The model under review builds one solid part; all positions refer to its coordinate system, in mm. A direction names the side the tool comes from. Coordinates: 2 decimals unless noted, no trailing zeros. Order: outer loops, then holes, each group sorted by start corner. A loop starts at its lowest first (then second) coordinate and runs counter-clockwise, first axis right, second up. Notation, with made-up numbers: M -34.5,-22 L -25.5,-22 A8 cw -25.5,-16 Z; hole C 26.5,67.5 d3. An arc over 180 degrees is marked long. Answer in a Markdown table with one row per item.
Autodesk Inventor part; units mm, degrees
ref_plane "YZ Plane" through (0, 0, 0) normal (1, 0, 0) x (0, 1, 0)
ref_plane "XZ Plane" through (0, 0, 0) normal (0, 1, 0) x (-1, 0, 0)
ref_plane "XY Plane" through (0, 0, 0) normal (0, 0, 1) x (1, 0, 0)
sketch "Boceto1" plane through (0, 0, 0) normal (0, 1, 0) x (-1, 0, 0)
  circle A0 centre (0, 0) radius 1.7
  line L0 (-10, -3) -> (10, -3)
  line L1 (10, -3) -> (10, 3)
  line L2 (10, 3) -> (-10, 3)
  line L3 (-10, 3) -> (-10, -3)
  line L4 (-10, -3) -> (10, 3) construction
  line L5 (10, -3) -> (-10, 3) construction
  line L6 (10, 3) -> (-10, 3)
  line L7 (-10, 3) -> (-10, 6)
  line L8 (-10, 6) -> (10, 6)
  line L9 (10, 6) -> (10, 3)
  line L10 (10, -3) -> (-10, -3)
  line L11 (-10, -3) -> (-10, -6)
  line L12 (-10, -6) -> (10, -6)
  line L13 (10, -6) -> (10, -3)
  dimension "d0" = 3.4
  dimension "d1" = 20
  dimension "d2" = 6
  dimension "d3" = 3
  dimension "d4" = 3
extrude "Extrusión1" add sketch "Boceto1" against normal blind 2 contours L3 L2 L1 L0
extrude "Extrusión2" add sketch "Boceto1" along normal blind 23 contours L0 L13 L12 L11 | L7 L8 L9 L2
sketch "Boceto2" plane through (-10, 0, 6) normal (0, 0, 1) x (1, 0, 0)
  line L0 (0, 0) -> (20, 0)
  line L1 (20, 0) -> (20, 23)
  line L2 (0, 23) -> (20, 23)
  line L3 (0, 0) -> (0, 23)
  circle A0 centre (17.46, 2.54) radius 1.2989
  circle A1 centre (17.46, 19.54) radius 1.2989
  circle A2 centre (4.86, 2.54) radius 1.2989
  circle A3 centre (4.86, 19.54) radius 1.2989
  point P0 (10, 0)
  dimension "d9" = 2.54
  dimension "d10" = 2.54
  dimension "d13" = 17
  dimension "d16" = 12.6
extrude "Extrusión3" cut sketch "Boceto2" against normal up to surface (3 mm away) contours A1 | A2
extrude "Extrusión4" add sketch "Boceto1" against normal blind 2 contours L0 L13 L12 L11 | L7 L8 L9 L2
extrude "Extrusión5" cut sketch "Boceto2" along normal up to surface (3 mm away) from surface at -12 contours A0 | A3
fillet "Empalme1" radius 3.5 4 edges at (-10, 23, 4.5) (-10, 23, -4.5) (10, 23, -4.5) (10, 23, 4.5)
properties part number "Sujetador_radar"
(1) The part is to be moulded in two halves that separate along Z. For faces 1 (the cylindrical face through (9, 21.95, 4.52)), 2 (the flat face through (0, 11, -6)), 3 (the flat face through (0, 11, 6)), 4 (the flat face through (0, 0, 2)), say which applies: +Z half, -Z half, draft (parallel to the pull), parting line (faces both ways), or undercut.
Report:
| item | result |
|---|---|
| face 1 | draft |
| face 2 | -Z half |
| face 3 | +Z half |
| face 4 | undercut |
(2) Take a section at D-D (y = 2.54). Write out the cut boundary in (x, z), then the cut area to 3 significant figures.
Report:
| item | result |
|---|---|
| outline | M -10,-6 L 6.16,-6 L 6.16,-3 L -10,-3 Z; M -10,3 L -6.44,3 L -6.44,6 L -10,6 Z; M -3.84,3 L 10,3 L 10,6 L -3.84,6 Z; M 8.76,-6 L 10,-6 L 10,-3 L 8.76,-3 Z |
| area | 104 mm^2 |
(3) Take a section at B-B (y = 7). Write out the cut boundary in (x, z).
Report:
| item | result |
|---|---|
| outline | M -10,-6 L 10,-6 L 10,-3 L -10,-3 Z; M -10,3 L 10,3 L 10,6 L -10,6 Z |
(4) To check wall thickness, follow line 1 (Z direction, x = 1.5, y = 21.5); line 2 (Y direction, x = -5.14, z = -5.15); line 3 (Y direction, x = -7, z = -2.25). State the ranges of each line that lie inside material, in increasing order. Write a range as [from, to].
Report:
| item | result |
|---|---|
| line 1 | [-6, -3], [3, 6] |
| line 2 | [-2, 18.24], [20.84, 23] |
| line 3 | [-2, 0] |
(5) Take a section at C-C (x = -5.14). Write out the cut boundary in (y, z), then the cut area to 3 significant figures.
Report:
| item | result |
|---|---|
| outline | M -2,-6 L 18.24,-6 L 18.24,-3 L 0,-3 L 0,3 L 1.24,3 L 1.24,6 L -2,6 Z; M 3.84,3 L 23,3 L 23,6 L 3.84,6 Z; M 20.84,-6 L 23,-6 L 23,-3 L 20.84,-3 Z |
| area | 146 mm^2 |
(6) Take a section at A-A (z = 0). Write out the cut boundary in (x, y).
Report:
| item | result |
|---|---|
| outline | M -10,-2 L -1.7,-2 L -1.7,0 L -10,0 Z; M 1.7,-2 L 10,-2 L 10,0 L 1.7,0 Z |
(7) Insertion check: P1, Ø2, axis at x = 7.46, y = 19.54, coming from the +Z side; P2, Ø3, axis at y = 5, z = -1, coming from the +X side. Each pin has a flat end and moves straight along its axis. Give the tip position at first contact, or say it passes through.
Report:
| item | result |
|---|---|
| P1 | z = -3 |
| P2 | through |
(8) Machinability: for faces 5 (the cylindrical face through (-3.9, 2.93, 4.52)), 6 (the cylindrical face through (6.43, 3.33, -4.52)), 7 (the flat face through (0, 11, -3)), 8 (the cylindrical face through (-9, 21.95, 4.48)), which of the approach directions +Z, -Z, +X, -X, +Y, -Y give a long, thin tool a straight path to every point of the face, cutting with its end or side? Answer none if there is none.
Report:
| item | result |
|---|---|
| face 5 | +Z |
| face 6 | -Z |
| face 7 | +X, -X, +Y |
| face 8 | +Z, -Z, -X, +Y |
